Here's how the part is built. I have some questions about the finished solid (model axes, mm). Face numbers are marked on the shaded views. A direction names the side the tool comes from. Give positions to 0.01 mm unless a question says otherwise; leave off trailing zeros. Write each loop counter-clockwise with the first axis right and the second up, starting at its lowest first coordinate (ties: lowest second). Pieces come first, ordered by that corner, then holes. Notation, with made-up numbers: (-33, 68) - (25, 68) arc R10 ccw to (25, 74) - close; hole circle Ø10 at (79.25, 20). An arc over 180 degrees is marked (long way). Write each question's results on one line, items separated by ' | '. Start each with the question number.
Item 1: We'd pull the mould along Z, two halves only. Please class the marked faces 4, 5 and 6: +Z half, -Z half, draft (parallel to the pull), parting line (faces both ways), or undercut.
Item 2: Suppose I cut it at C-C on z = 22.5. List the corners of the cut face in (x, y) for me.
Item 3: Which directions (+Z, -Z, +X, -X, +Y, -Y) give clear straight access to the entire face, cutting with the end or side of a thin tool? Please do the marked faces 1, 2 and 3.
Item 4: Suppose I cut it at D-D on x = -59. List the corners of the cut face in (y, z) for me.
Item 5: Suppose I cut it at B-B on y = -90. List the corners of the cut face in (x, z) for me.
Item 6: Will these pins go through, and if not, where does the flat tip stop? P1, Ø4, axis at x = 2.5, y = -45.5, coming from the +Z side; P2, Ø16, axis at x = -63, y = -141.5, coming from the +Z side; P3, Ø11.5, axis at x = 0, y = -50, coming from the -Z side.
Item 7: Please list where these lines run through material, in increasing order: line 1 along Y through (x, z) = (0, -68); line 2 along X through (y, z) = (-12, -88.5); line 3 along Y through (x, z) = (-1, -64).
Item 8: Suppose I cut it at A-A on x = 16. List the corners of the cut face in (y, z) for me, then the cut area to 3 significant figures.
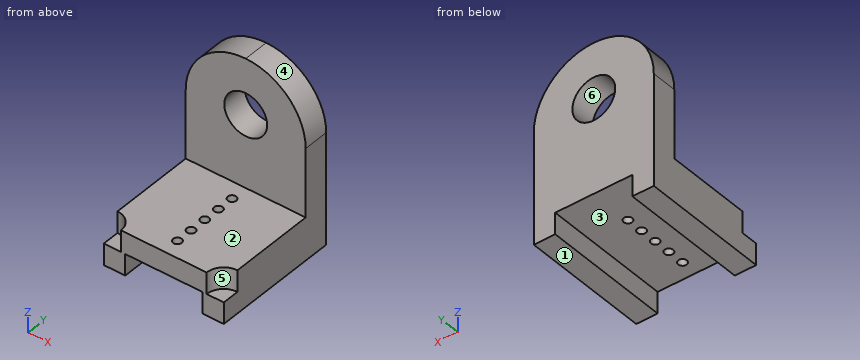
```python
from build123d import *

# Parameters (mm, degrees)
F0_W      = 140
F0_H      = 175
F1_DEPTH  = 30
F2_R      = 69.99999
F3_R      = 25
F4_DEPTH  = 30.001
F5_W      = 140
F5_H      = 25
F6_DEPTH  = 120
F7_W      = 25
F7_H      = 150
F8_DEPTH  = 25
F9_R      = 20
F10_DEPTH = 25
F11_R     = 5
F12_DEPTH = 50.001


# Not quite as in the source:
# - a fillet or chamfer is up to 0.001 mm smaller than in the source, because OpenCascade refuses the exact size


with BuildPart() as f1:
    # F0 (on Front) → F1 (new body)
    with BuildSketch(Plane.XZ):
        Rectangle(F0_W, F0_H)
    extrude(amount=F1_DEPTH)

    # F2 (radius 70 in the source; OpenCascade refuses exactly that, so slightly less here)
    f2_edges = [f1.edges().sort_by_distance(p)[0] for p in [
        (70, -15, 87.5),
        (-70, -15, 87.5),
    ]]
    fillet(f2_edges, radius=F2_R)

    # F3 (on face) → F4 (cut, through all)
    with BuildSketch(Plane.XZ.offset(30)):
        with Locations((0, 22.5)):
            Circle(F3_R)
    extrude(amount=-F4_DEPTH, mode=Mode.SUBTRACT)

    # F5 (on face) → F6 (join)
    with BuildSketch(Plane.XZ.offset(30)):
        with Locations((0, -75)):
            Rectangle(F5_W, F5_H)
    extrude(amount=F6_DEPTH)

    # F7 (on face) → F8 (join)
    with BuildSketch(Plane(origin=(0, 0, -87.5), x_dir=(1, 0, 0), z_dir=(0, 0, -1))):
        with Locations((-57.5, 75)):
            Rectangle(F7_W, F7_H)
        with Locations((57.5, 75)):
            Rectangle(F7_W, F7_H)
    extrude(amount=F8_DEPTH)

    # F9 (on face) → F10 (cut)
    with BuildSketch(Plane.XY.offset(-62.5)):
        with Locations((-70, -150)):
            Circle(F9_R)
        with Locations((70, -150)):
            Circle(F9_R)
    extrude(amount=-F10_DEPTH, mode=Mode.SUBTRACT)

    # F11 (on face) → F12 (cut, through all)
    with BuildSketch(Plane.XY.offset(-62.5)):
        with Locations((0, -130)):
            Circle(F11_R)
        with Locations((0, -110)):
            Circle(F11_R)
        with Locations((0, -90)):
            Circle(F11_R)
        with Locations((0, -70)):
            Circle(F11_R)
        with Locations((0, -50)):
            Circle(F11_R)
    extrude(amount=-F12_DEPTH, mode=Mode.SUBTRACT)


solid = f1.part
```
Checked values:
1) face 4: +Z half | face 5: draft | face 6: undercut
2) outline: (-69.82, -30) - (-25, -30) - (-25, 0) - (-69.82, 0) - close; (25, -30) - (69.82, -30) - (69.82, 0) - (25, 0) - close
3) face 1: -Z, +X, -X, +Y, -Y | face 2: +Z, +X, -X, -Y | face 3: -Z, +Y, -Y
4) outline: (-150, -112.5) - (0, -112.5) - (0, 55.17) - (-30, 55.17) - (-30, -62.5) - (-133.3, -62.5) - (-133.3, -87.5) - (-150, -87.5) - close
5) outline: (-70, -112.5) - (-45, -112.5) - (-45, -87.5) - (-5, -87.5) - (-5, -62.5) - (-70, -62.5) - close; (5, -87.5) - (45, -87.5) - (45, -112.5) - (70, -112.5) - (70, -62.5) - (5, -62.5) - close
6) P1: stops at z = -62.5 | P2: stops at z = -87.5 | P3: stops at z = -87.5
7) line 1: y = -150 to -135, -125 to -115, -105 to -95, -85 to -75, -65 to -55, -45 to 0 | line 2: x = -70 to -45, 45 to 70 | line 3: y = -150 to -134.9, -125.1 to -114.9, -105.1 to -94.9, -85.1 to -74.9, -65.1 to -54.9, -45.1 to 0
8) outline: (-150, -87.5) - (0, -87.5) - (0, 3.29) - (-30, 3.29) - (-30, -62.5) - (-150, -62.5) - close; (-30, 41.71) - (0, 41.71) - (0, 85.65) - (-30, 85.65) - close | area: 7,040 mm^2
